For this review, take the finished solid that the model builds, in its own axes (mm). Face numbers are marked on the shaded views. A direction names the side the tool comes from. Give positions to 0.01 mm unless a question says otherwise; leave off trailing zeros. Order: outer loops, then holes, each group sorted by start corner. A loop starts at its lowest first (then second) coordinate and runs counter-clockwise, first axis right, second up. Notation, with made-up numbers: M -22.75,-4 L -14.75,-4 A24 cw -14.75,32 Z; hole C 38.25,20 d11. An arc over 180 degrees is marked long. Use CSV: the item, a comma, the result in double quotes. Start each with the question number.
(1) Tool access review of the marked faces 1 and 2: name each direction out of +Z, -Z, +X, -X, +Y, -Y from which nothing blocks a thin tool from reaching the whole face with its end or side.
(2) Clearance check with flat-ended pins moving along their axes: P1, Ø6, axis at x = -81.5, z = 12.5, coming from the +Y side; P2, Ø9.5, axis at y = 33.46, z = -20.14, coming from the -X side; P3, Ø0.6, axis at x = -63.5, y = 1.5, coming from the +Z side; P4, Ø2, axis at x = -59.5, z = 3, coming from the +Y side. State where each tip first meets the part, or that it passes through.
(3) Consider section D-D (z = -24.5). Write out the cut boundary in (x, y).
(4) Consider section C-C (z = -14). Write out the cut boundary in (x, y).
(5) Consider section A-A (x = -58.5). Write out the cut boundary in (y, z), and give its area (3 significant figures).
(6) Consider section B-B (y = 14.5). Write out the cut boundary in (x, z), and give its area (3 significant figures).
(7) Wall thickness on L1, parallel to X at y = 13, z = -11; L2, parallel to Y at x = -48, z = -21: over which ranges is each line inside the solid? List them lowest first. Write a range as from..to.
```python
from build123d import *

# Parameters (mm, degrees)
SKETCH017_W  = 42
SKETCH017_H  = 45
SKETCH017_R  = 3
PAD012_DEPTH = 2
SKETCH018_W  = 57.5
SKETCH018_H  = 45
PAD013_DEPTH = 2
FILLET_R     = 22


with BuildPart() as part:
    # Sketch017 → Pad012 (new body)
    with BuildSketch(Plane(origin=(-40, 3, -3), x_dir=(0, 1, 0), z_dir=(1, 0, 0))):
        with Locations((18.460948, -2.635084)):
            Rectangle(SKETCH017_W, SKETCH017_H)
        with Locations((12.460948, 11.864916)):
            Circle(SKETCH017_R, mode=Mode.SUBTRACT)
        with Locations((30.460948, 11.864916)):
            Circle(SKETCH017_R, mode=Mode.SUBTRACT)
        with Locations((30.460948, -17.135084)):
            Circle(SKETCH017_R, mode=Mode.SUBTRACT)
        with Locations((12.460948, -17.135084)):
            Circle(SKETCH017_R, mode=Mode.SUBTRACT)
    extrude(amount=-PAD012_DEPTH)

    # Sketch018 → Pad013 (join)
    with BuildSketch(Plane(origin=(-21, 0, -3), x_dir=(1, 0, 0), z_dir=(0, -1, 0))):
        with Locations((-49.725473, -2.637928)):
            Rectangle(SKETCH018_W, SKETCH018_H)
        with BuildLine():
            Line((-57, -15), (-45, -15))
            ThreePointArc((-45, -15), (-36.161165, -11.338835), (-32.5, -2.5))
            Line((-32.5, -2.5), (-32.5, -1.5))
            ThreePointArc((-32.5, -1.5), (-36.161165, 7.338835), (-45, 11))
            Line((-45, 11), (-57, 11))
            ThreePointArc((-57, 11), (-65.838835, 7.338835), (-69.5, -1.5))
            Line((-69.5, -1.5), (-69.5, -2.5))
            ThreePointArc((-69.5, -2.5), (-65.838835, -11.338835), (-57, -15))
        make_face(mode=Mode.SUBTRACT)
    extrude(amount=-PAD013_DEPTH)

    # Fillet
    fillet_edges = [part.edges().sort_by_distance(p)[0] for p in [
        (-99.475473, 1, -28.137928),
        (-99.475473, 1, 16.862072),
    ]]
    fillet(fillet_edges, radius=FILLET_R)


solid = part.part
```
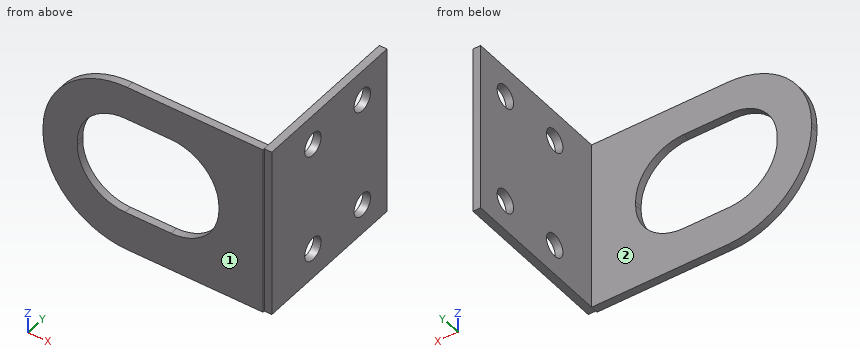
Check result:
1,face 1,"+Z, -Z, +X, -X, -Y"
1,face 2,"+Z, -Z, -X, +Y"
2,P1,"stops at y = 2"
2,P2,"stops at x = -42"
2,P3,"stops at z = 16.86"
2,P4,"passes through"
3,outline,"M -89.59,0 L -41.98,0 L -41.98,0.46 L -40,0.46 L -40,42.46 L -42,42.46 L -42,2 L -89.59,2 Z"
4,outline,"M -98.02,0 L -87.17,0 L -87.17,2 L -98.02,2 Z; M -56.83,0 L -41.98,0 L -41.98,0.46 L -40,0.46 L -40,42.46 L -42,42.46 L -42,2 L -56.83,2 Z"
5,outline,"M 0,-28.14 L 2,-28.14 L 2,-15.5 L 0,-15.5 Z; M 0,5.5 L 2,5.5 L 2,16.86 L 0,16.86 Z"
5,area,"48.0 mm^2"
6,outline,"M -42,-28.14 L -40,-28.14 L -40,-22.98 L -42,-22.98 Z; M -42,-17.29 L -40,-17.29 L -40,6.02 L -42,6.02 Z; M -42,11.71 L -40,11.71 L -40,16.86 L -42,16.86 Z"
6,area,"67.3 mm^2"
7,L1,"x = -42..-40"
7,L2,"y = 0..2"
